from build123d import *

# Parameters (mm, degrees)
LPATTERN1_COUNT          = 7
LPATTERN1_PITCH          = 24
LPATTERN2_COUNT          = 2
LPATTERN2_PITCH          = 24
BOSS_EXTRUDE1_REACH      = 175.781
SKETCH4_W                = 24
SKETCH4_H                = 10
SKETCH5_W                = 10
SKETCH5_H                = 10
BOSS_EXTRUDE2_DEPTH      = 10
CUT_EXTRUDE1_DEPTH       = 10
CHAMFER3_SIZE            = 2
CHAMFER3_OF_MIRROR2_SIZE = 2


with BuildPart() as part:
    # Sketch1 → Revolve1 (revolve)
    with BuildSketch(Plane(origin=(0, 0, 0), x_dir=(0, 0, -1), z_dir=(1, 0, 0))):
        Polygon((-12.875, 5), (-12.875, -5), (-6, -5), (-6, -3), (-10.875, -3), (-10.875, 5), align=None)
    revolve1 = revolve(axis=Axis((0, 27.077205882, 0), (0, -1, 0)))

    # LPattern1: Revolve1 ×7
    with Locations(*[(0, 0, -i * LPATTERN1_PITCH) for i in range(1, LPATTERN1_COUNT)]):
        add(revolve1)

    # LPattern2: Revolve1 ×2
    with Locations(*[(i * LPATTERN2_PITCH, 0, 0) for i in range(1, LPATTERN2_COUNT)]):
        add(revolve1)

    # LPattern2 copy 1 sketch → LPattern2 copy 1 (revolve)
    with BuildSketch(Plane(origin=(24, 0, -24), x_dir=(0, 0, -1), z_dir=(1, 0, 0))):
        Polygon((-12.875, 5), (-12.875, -5), (-6, -5), (-6, -3), (-10.875, -3), (-10.875, 5), align=None)
    revolve(axis=Axis((24, 27.077205882, -24), (0, -1, 0)))

    # LPattern2 copy 2 sketch → LPattern2 copy 2 (revolve)
    with BuildSketch(Plane(origin=(24, 0, -48), x_dir=(0, 0, -1), z_dir=(1, 0, 0))):
        Polygon((-12.875, 5), (-12.875, -5), (-6, -5), (-6, -3), (-10.875, -3), (-10.875, 5), align=None)
    revolve(axis=Axis((24, 27.077205882, -48), (0, -1, 0)))

    # LPattern2 copy 3 sketch → LPattern2 copy 3 (revolve)
    with BuildSketch(Plane(origin=(24, 0, -72), x_dir=(0, 0, -1), z_dir=(1, 0, 0))):
        Polygon((-12.875, 5), (-12.875, -5), (-6, -5), (-6, -3), (-10.875, -3), (-10.875, 5), align=None)
    revolve(axis=Axis((24, 27.077205882, -72), (0, -1, 0)))

    # LPattern2 copy 4 sketch → LPattern2 copy 4 (revolve)
    with BuildSketch(Plane(origin=(24, 0, -96), x_dir=(0, 0, -1), z_dir=(1, 0, 0))):
        Polygon((-12.875, 5), (-12.875, -5), (-6, -5), (-6, -3), (-10.875, -3), (-10.875, 5), align=None)
    revolve(axis=Axis((24, 27.077205882, -96), (0, -1, 0)))

    # LPattern2 copy 5 sketch → LPattern2 copy 5 (revolve)
    with BuildSketch(Plane(origin=(24, 0, -120), x_dir=(0, 0, -1), z_dir=(1, 0, 0))):
        Polygon((-12.875, 5), (-12.875, -5), (-6, -5), (-6, -3), (-10.875, -3), (-10.875, 5), align=None)
    revolve(axis=Axis((24, 27.077205882, -120), (0, -1, 0)))

    # LPattern2 copy 6 sketch → LPattern2 copy 6 (revolve)
    with BuildSketch(Plane(origin=(24, 0, -144), x_dir=(0, 0, -1), z_dir=(1, 0, 0))):
        Polygon((-12.875, 5), (-12.875, -5), (-6, -5), (-6, -3), (-10.875, -3), (-10.875, 5), align=None)
    revolve(axis=Axis((24, 27.077205882, -144), (0, -1, 0)))

    # Sketch4 → Boss-Extrude1 (add, up to next)
    with BuildSketch(Plane.XY.offset(12.875), mode=Mode.PRIVATE) as boss_extrude1_sk1:
        with Locations((12, 0)):
            Rectangle(SKETCH4_W, SKETCH4_H)
    boss_extrude1_tool1 = extrude(boss_extrude1_sk1.sketch, amount=-BOSS_EXTRUDE1_REACH, mode=Mode.PRIVATE) - part.part
    boss_extrude1 = boss_extrude1_tool1.solids().sort_by_distance((12, 0, 12.875))[0]
    add(boss_extrude1)

    # Sketch5 → Boss-Extrude2 (add)
    with BuildSketch(Plane.XY.offset(12.875)):
        with Locations((12, 0)):
            Rectangle(SKETCH5_W, SKETCH5_H)
    boss_extrude2 = extrude(amount=BOSS_EXTRUDE2_DEPTH)

    # Sketch8 → Cut-Extrude1 (cut)
    with BuildSketch(Plane.ZY.offset(-7)):
        Polygon((19.895725942, -3.5), (21.916451884, 0), (19.895725942, 3.5), (15.854274058, 3.5), (13.833548116, 0), (15.854274058, -3.5), align=None)
    cut_extrude1 = extrude(amount=-CUT_EXTRUDE1_DEPTH, mode=Mode.SUBTRACT)

    # Chamfer3
    chamfer3_edges = [part.edges().sort_by_distance(p)[0] for p in [
        (12, -5, 22.875),
        (12, 5, 22.875),
    ]]
    chamfer(chamfer3_edges, length=CHAMFER3_SIZE)

    # Mirror2: Boss-Extrude1, Boss-Extrude2, Cut-Extrude1 across plane
    add(boss_extrude1.mirror(Plane.XY.offset(-72)))
    add(boss_extrude2.mirror(Plane.XY.offset(-72)))
    add(cut_extrude1.mirror(Plane.XY.offset(-72)), mode=Mode.SUBTRACT)

    # Chamfer3 of Mirror2
    chamfer3_of_mirror2_edges = [part.edges().sort_by_distance(p)[0] for p in [
        (12, -5, -166.875),
        (12, 5, -166.875),
    ]]
    chamfer(chamfer3_of_mirror2_edges, length=CHAMFER3_OF_MIRROR2_SIZE)


solid = part.part
The model under review builds one solid part; all positions refer to its coordinate system, in mm. A direction names the side the tool comes from. Coordinates: 2 decimals unless noted, no trailing zeros. Write each loop counter-clockwise with the first axis right and the second up, starting at its lowest first coordinate (ties: lowest second). Pieces come first, ordered by that corner, then holes. Notation, with made-up numbers: (-2, -26.75) -> (37, -26.75) arc R19 ccw to (37, -1.75) -> close; hole circle Ø7 at (64, 2). An arc over 180 degrees is marked (long way). Answer in a Markdown table with one row per item.
1. Clearance check with flat-ended pins moving along their axes: pin 1 Ø2 at (x, y) = (20.5, 0) entering from -Z (3 decimals); pin 2 Ø17.5 at (x, z) = (23.5, -98) entering from +Y; pin 3 Ø5 at (y, z) = (0.5, -33) entering from +X. State where each tip first meets the part, or that it passes through.
Answers below:
| item | result |
|---|---|
| pin 1 | stops at z = -156.875 |
| pin 2 | stops at y = -3 |
| pin 3 | stops at x = 35.11 |
2. For faces 1 (the flat face through (5, -3, -125)), 2 (the flat face through (20, 0, -156.875)), 3 (the cylindrical face through (27.65, -3.99, -28.76)), 4 (the flat face through (11.93, -1.726, -158.83)), list the 3-axis set-ups (+Z, -Z, +X, -X, +Y, -Y) from which the entire face can be reached by the end or side of a thin tool; tool diameter is ignored.
Answers below:
| item | result |
|---|---|
| face 1 | +Y |
| face 2 | -Z, +X, +Y, -Y |
| face 3 | +Y, -Y |
| face 4 | +X, -X |
3. We need section A-A, the plane z = -48. State the section outline as (x, y) points (3 decimals).
Answers below:
| item | result |
|---|---|
| outline | (-12.875, -5) -> (-6, -5) -> (-6, -3) -> (-10.875, -3) -> (-10.875, 5) -> (-12.875, 5) -> close; (6, -5) -> (18, -5) -> (18, -3) -> (13.125, -3) -> (13.125, 5) -> (10.875, 5) -> (10.875, -3) -> (6, -3) -> close; (30, -5) -> (36.875, -5) -> (36.875, 5) -> (34.875, 5) -> (34.875, -3) -> (30, -3) -> close |
4. Draft analysis for pull direction X (two halves, no side actions). For faces 5 (the flat face through (3, 0, -156.875)), 6 (the flat face through (5, -3, -149)), 7 (the cylindrical face through (0, -4, -6)), state which applies: +X half, -X half, draft (parallel to the pull), parting line (faces both ways), or undercut.
Answers below:
| item | result |
|---|---|
| face 5 | draft |
| face 6 | undercut |
| face 7 | undercut |
5. Wall thickness on probe 1 along X at (y, z) = (2, -152); probe 2 along X at (y, z) = (-2, -148.5); probe 3 along X at (y, z) = (-0.75, -62): over which ranges is each line inside the solid? List them lowest first. Write a range as [from, to].
Answers below:
| item | result |
|---|---|
| probe 1 | x = [-10.09, -7.37], [7.37, 16.63], [31.37, 34.09] |
| probe 2 | x = [-12.06, -9.9], [9.9, 14.1], [33.9, 36.06] |
| probe 3 | x = [-8.11, -4.27], [4.27, 8.11], [15.89, 19.73], [28.27, 32.11] |
